Autodesk Fusion 360 part; units mm, degrees
sketch "Sketch1" plane through (0, 0, 0) normal (0, 0, 1) x (1, 0, 0)
  line L0 (-75, 50) -> (75, 50)
  line L1 (75, 50) -> (75, -50)
  line L2 (75, -50) -> (-75, -50)
  line L3 (-75, -50) -> (-75, 50)
  line L4 (-75, 50) -> (75, -50) construction
  line L5 (75, 50) -> (-75, -50) construction
  dimension "d1" = 150
  dimension "d2" = 100
extrude "Extrude1" add sketch "Sketch1" along normal blind 20
sketch "Sketch2" plane through (0, 0, 20) normal (0, 0, 1) x (-1, 0, 0)
  line L0 (75, 50) -> (-75, 50)
  line L1 (-75, 50) -> (-75, -50)
  line L2 (-75, -50) -> (75, -50)
  line L3 (75, -50) -> (75, 50)
  circle A0 centre (0, 0) radius 40
  dimension "d5" = 80
extrude "Extrude2" add sketch "Sketch2" along normal blind 40 contours A0
fillet "Fillet1" radius 40 1 edges at (37.2931, 14.4646, 60)
Design review of the part built by this model. Coordinates are the model's own, in mm. Round coordinates to 2 decimals unless told otherwise and drop trailing zeros. Write each loop counter-clockwise with the first axis right and the second up, starting at its lowest first coordinate (ties: lowest second). Pieces come first, ordered by that corner, then holes. Notation, with made-up numbers: (55, 18.25) - (114, 18.25) arc R36 ccw to (114, 54.25) - close; hole circle Ø2 at (25.5, -23.5). An arc over 180 degrees is marked (long way). Use a Markdown table: item, result. Add a question column.
1. We need section A-A (x = 50.5). State the section outline as (y, z) points.
2. Clearance check with flat-ended pins moving along their axes: pin 1 (4 mm diameter, centred on x = 57.5, y = -12.5, fed in from +Z); pin 2 (4 mm diameter, centred on x = 33.5, y = -16.5, fed in from +Z); pin 3 (1.5 mm diameter, centred on x = -8, z = 52, fed in from +Y). State where each tip first meets the part, or that it passes through.
3. Wall thickness on probe 1 along Z at (x, y) = (-14, 45.5); probe 2 along Z at (x, y) = (7.5, 9.5); probe 3 along X at (y, z) = (14, 41): over which ranges is each line inside the solid? List them lowest first.
4. Mouldability with a two-part tool opening along Y and no side actions: class faces 1 (the face through (-1, 50, 10)), 2 (the face through (1, -50, 10)), 3 (the face through (-34, -22, 20)) as +Y half, -Y half, draft (parallel to the pull), parting line (faces both ways), or undercut.
Output:
| question | item | result |
|---|---|---|
| 1 | outline | (-50, 0) - (50, 0) - (50, 20) - (-50, 20) - close |
| 2 | pin 1 | stops at z = 20 |
| 2 | pin 2 | stops at z = 38.74 |
| 2 | pin 3 | stops at y = 23.69 |
| 3 | probe 1 | z = 0 to 20 |
| 3 | probe 2 | z = 0 to 58.13 |
| 3 | probe 3 | x = -31.04 to 31.04 |
| 4 | face 1 | +Y half |
| 4 | face 2 | -Y half |
| 4 | face 3 | draft |
